For this review, take the finished solid that the model builds, in its own axes (mm). Face numbers are marked on the shaded views. Round coordinates to 2 decimals unless told otherwise and drop trailing zeros. Loops run counter-clockwise (first coordinate to the right, second up) from the corner with the lowest first, then second, coordinate; pieces in that order, holes last. Notation, with made-up numbers: M -21.5,35 L 0.5,35 A27 cw 0.5,56 Z; hole C -40,36.5 d9. An arc over 180 degrees is marked long. Write item = value, one per line. Start each with the question number.
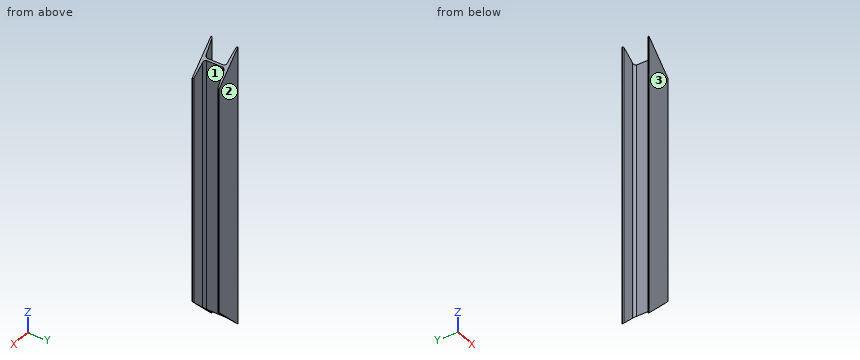
Autodesk Inventor part; units mm, degrees
ref_plane "Начальная плоскость" through (0, 0, -70) normal (0, 0, 1) x (1, 0, 0)
ref_plane "Конечная плоскость" through (0, 0, 1370) normal (0, 0, 1) x (1, 0, 0)
ref_plane "РабПлоскость4" through (-70, 0, 1370) normal (0.7071, 0, 0.7071) x (0.7071, 0, -0.7071)
ref_plane "Начальная плоскость" through (0, 0, -70) normal (0, 0, 1) x (1, 0, 0)
ref_plane "Конечная плоскость" through (0, 0, 1370) normal (0, 0, 1) x (1, 0, 0)
sketch "Эскиз" plane through (0, 0, 0) normal (0, 0, 1) x (1, 0, 0)
  line L0 (-3.5, 0) -> (-3.5, -42.8956)
  line L1 (-13.8299, -54.7788) -> (-64.835, -61.9471)
  line L2 (-70, -67.8887) -> (-70, -70)
  line L3 (-70, -70) -> (0, -70)
  line L4 (-36.75, -70) -> (-36.75, -58) construction
  line L5 (-61.3329, 0) -> (81.7772, 0) construction
  line L6 (0, 0) -> (0, -70) construction
  line L7 (0, -60) -> (0, 80) construction
  line L8 (3.5, 0) -> (3.5, -42.8956)
  line L9 (13.8299, -54.7788) -> (64.835, -61.9471)
  line L10 (70, -67.8887) -> (70, -70)
  line L11 (70, -70) -> (0, -70)
  line L12 (-3.5, 0) -> (0, 0) construction
  line L13 (-3.5, 0) -> (-3.5, 42.8956)
  line L14 (-13.8299, 54.7788) -> (-64.835, 61.9471)
  line L15 (-70, 67.8887) -> (-70, 70)
  line L16 (-70, 70) -> (0, 70)
  line L17 (3.5, 0) -> (3.5, 42.8956)
  line L18 (13.8299, 54.7788) -> (64.835, 61.9471)
  line L19 (70, 67.8887) -> (70, 70)
  line L20 (70, 70) -> (0, 70)
  arc A0 (-70, 67.8887) -> (-64.835, 61.9471) centre (-64, 67.8887) ccw
  arc A1 (64.835, 61.9471) -> (70, 67.8887) centre (64, 67.8887) ccw
  arc A2 (70, -67.8887) -> (64.835, -61.9471) centre (64, -67.8887) ccw
  arc A3 (-64.835, -61.9471) -> (-70, -67.8887) centre (-64, -67.8887) ccw
  arc A4 (-3.5, 42.8956) -> (-13.8299, 54.7788) centre (-15.5, 42.8956) ccw
  arc A5 (13.8299, 54.7788) -> (3.5, 42.8956) centre (15.5, 42.8956) ccw
  arc A6 (3.5, -42.8956) -> (13.8299, -54.7788) centre (15.5, -42.8956) ccw
  arc A7 (-13.8299, -54.7788) -> (-3.5, -42.8956) centre (-15.5, -42.8956) ccw
  line L21 (0, 110) -> (0, -100) construction
  line L22 (-101.6883, 0) -> (112.3548, 0) construction
  point P0 (-3.5, -53.327)
  point P1 (-70, -62.673)
  point P2 (3.5, -53.327)
  point P3 (70, -62.673)
  point P4 (36.75, -70)
  point P5 (36.75, -58)
  point P6 (-3.5, 53.327)
  point P7 (-70, 62.673)
  point P8 (-36.75, 70)
  point P9 (-36.75, 58)
  point P10 (3.5, 53.327)
  point P11 (70, 62.673)
  point P12 (36.75, 58)
  point P13 (36.75, 70)
  dimension "d1" = 12
  dimension "d2" = 33.25
  dimension "d3" = 3.5
  dimension "d4" = 70
  dimension "d9" = 70
  dimension "d14" = 98
  dimension "d15" = 6
  dimension "d16" = 12
extrude "Тело" add sketch "Эскиз" along normal up to surface (1440 mm away) from surface at -70
sketch "Sketch3" plane through (0, 0, 0) normal (0, 0, 1) x (1, 0, 0)
  line L0 (0, 0) -> (10, 0)
ref_plane "Work Plane3" through (0, 0, 0) normal (0, -1, 0) x (1, 0, 0)
sketch "Sketch4" plane through (0, 0, 0) normal (0, -1, 0) x (1, 0, 0)
  line L0 (-2, -70) -> (12, -70)
  line L1 (-2, 1370) -> (12, 1370)
  dimension "d20" = 1440
ref_plane "РабПлоскость4" through (-70, 0, 1370) normal (0.7071, 0, 0.7071) x (0.7071, 0, -0.7071)
split "Разделение1" plane through (-70, 0, 1370) removes the side toward (0.7071, 0, 0.7071)
ref_plane "РабПлоскость5" through (-70, 0, -70) normal (0.7071, 0, -0.7071) x (-0.7071, 0, -0.7071)
split "Разделение2" plane through (-70, 0, -70) removes the side toward (0.7071, 0, -0.7071)
equation "\"d1\" = G_T1"
equation "\"d2\" = -0.25 * G_T + 0.25 * G_W"
equation "\"d3\" = 0.5 * G_T"
equation "\"d4\" = 0.5 * G_W"
equation "\"d9\" = 0.5 * G_H"
equation "\"d14\" = G_NG"
equation "\"d15\" = G_ER"
equation "\"d16\" = G_IR"
equation "\"d5\" = G_L"
equation "\"G_T\" = 7"
equation "\"G_T1\" = 12"
equation "\"G_L\" = d20"
equation "\"G_ER\" = 6"
equation "\"G_IR\" = 12"
equation "\"G_NG\" = 98deg"
properties part number "ISO 657 16 - SC 140 - 1440" material "Сталь, мягкая"
(1) Wall thickness on L1, parallel to Y at x = -13, z = 886; L2, parallel to X at y = 31, z = 799; L3, parallel to X at y = 63.5, z = 1207: over which ranges is each line inside the solid? List them lowest first.
(2) For pin 1 Ø2 at (y, z) = (3, 1051) entering from -X; pin 2 Ø5 at (y, z) = (0.5, 913) entering from +X, all flat-tipped, find the tip position at first contact; note any pin that passes through.
(3) Add section D-D on x = -38.5. Write out the cut boundary in (y, z).
(4) Add section B-B on x = 29. Write out the cut boundary in (y, z).
(5) Draft analysis for pull direction Y (two halves, no side actions). For the marked faces 1, 2 and 3, state which applies: +Y half, -Y half, draft (parallel to the pull), parting line (faces both ways), or undercut.
(6) Add section A-A on z = 298.5. Write out the cut boundary in (x, y) (3 decimals).
(7) Add section C-C on y = 21.5. Write out the cut boundary in (x, z), and give its area (3 significant figures).
Answer sheet:
q1.L1 = -70 to -54.63, 54.63 to 70
q1.L2 = -3.5 to 3.5
q1.L3 = -68.09 to 68.09
q2.pin_1 = -3.5
q2.pin_2 = 3.5
q3.outline = M -70,-38.5 L -58.25,-38.5 L -58.25,1338.5 L -70,1338.5 Z; M 58.25,-38.5 L 70,-38.5 L 70,1338.5 L 58.25,1338.5 Z
q4.outline = M -70,29 L -56.91,29 L -56.91,1271 L -70,1271 Z; M 56.91,29 L 70,29 L 70,1271 L 56.91,1271 Z
q5.face_1 = undercut
q5.face_2 = +Y half
q5.face_3 = -Y half
q6.outline = M -70,-70 L 70,-70 L 70,-67.889 A6 ccw 64.835,-61.947 L 13.83,-54.779 A12 cw 3.5,-42.896 L 3.5,42.896 A12 cw 13.83,54.779 L 64.835,61.947 A6 ccw 70,67.889 L 70,70 L -70,70 L -70,67.889 A6 ccw -64.835,61.947 L -13.83,54.779 A12 cw -3.5,42.896 L -3.5,-42.896 A12 cw -13.83,-54.779 L -64.835,-61.947 A6 ccw -70,-67.889 Z
q7.outline = M -3.5,-3.5 L 3.5,3.5 L 3.5,1296.5 L -3.5,1303.5 Z
q7.area = 9,100 mm²
